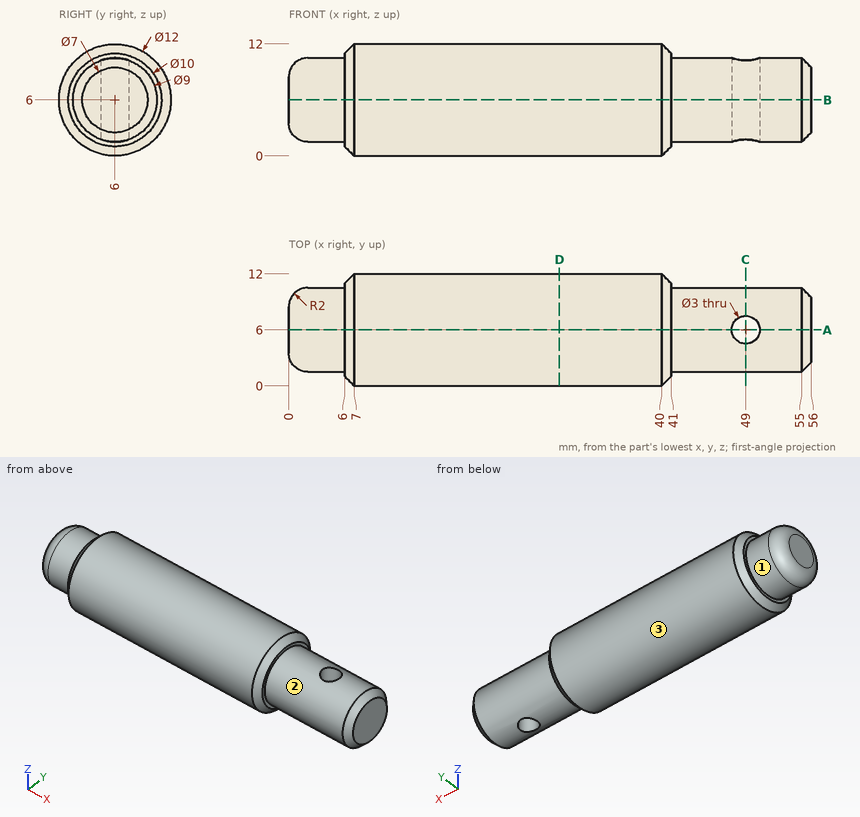
Check sheet for the drawn part. Datum: minimum x, y, z corner. Units: mm. A direction names the side the tool comes from. Round coordinates to 2 decimals unless told otherwise and drop trailing zeros. Order: outer loops, then holes, each group sorted by start corner. A loop starts at its lowest first (then second) coordinate and runs counter-clockwise, first axis right, second up.
1. Section check C-C on x = 49. Record the cut outline in (y, z).
Final values:
outline: (4.5, 1.76) - (4.5, 10.24) arc R4.5 ccw to start; (7.5, 1.76) arc R4.5 ccw to (7.5, 10.24) - close
2. Thickness scan on L1, parallel to X at y = 6, z = 8; L2, parallel to X at y = 5, z = 1.5; L3, parallel to Z at x = 24.5, y = 6.25. Record the ranges inside material, lowest first.
Final values:
L1: x = 0 to 47.5, 50.5 to 56
L2: x = 6 to 41
L3: z = 0.01 to 11.99
3. Access from +Z, -Z, +X, -X, +Y, -Y to the whole of each face (thin tool, end or side, straight path). Record for the marked faces 1, 2 and 3.
Final values:
face 1: -X
face 2: +X
face 3: +X, -X
4. Section check A-A on y = 6. Record the cut outline in (x, z), then the cut area to 3 significant figures.
Final values:
outline: (0, 3.5) arc R2 ccw to (2, 1.5) - (6, 1.5) - (6, 1) - (7, 0) - (40, 0) - (41, 1) - (41, 1.5) - (47.5, 1.5) - (47.5, 10.5) - (41, 10.5) - (41, 11) - (40, 12) - (7, 12) - (6, 11) - (6, 10.5) - (2, 10.5) arc R2 ccw to (0, 8.5) - close; (50.5, 1.5) - (55, 1.5) - (56, 2.5) - (56, 9.5) - (55, 10.5) - (50.5, 10.5) - close
area: 577 mm2
5. Section check B-B on z = 6. Record the cut outline in (x, y).
Final values:
outline: (0, 3.5) arc R2 ccw to (2, 1.5) - (6, 1.5) - (6, 1) - (7, 0) - (40, 0) - (41, 1) - (41, 1.5) - (55, 1.5) - (56, 2.5) - (56, 9.5) - (55, 10.5) - (41, 10.5) - (41, 11) - (40, 12) - (7, 12) - (6, 11) - (6, 10.5) - (2, 10.5) arc R2 ccw to (0, 8.5) - close; hole circle Ø3 at (49, 6)
6. Go/stop test with flat-tipped pins: P1, Ø2, axis at x = 27, z = 4, coming from the -Y side; P2, Ø1, axis at y = 2.5, z = 2.5, coming from the +X side; P3, Ø2, axis at x = 10.5, z = 4.5, coming from the -Y side; P4, Ø1.8, axis at x = 49, y = 6, coming from the +Z side (3 decimals). Record where each tip stops, or that it passes through.
Final values:
P1: stops at y = 0.08
P2: stops at x = 55.05
P3: stops at y = 0.02
P4: passes through
7. Section check D-D on x = 29. Record the cut outline in (y, z).
Final values:
outline: circle Ø12 at (6, 6)
